Source: CAD feature listing. Evaluate the final solid. Frame: model axes, mm. A direction names the side the tool comes from. Give positions to 0.01 mm unless a question says otherwise; leave off trailing zeros. Write each loop counter-clockwise with the first axis right and the second up, starting at its lowest first coordinate (ties: lowest second). Pieces come first, ordered by that corner, then holes. Notation, with made-up numbers: (-12.75, -19.5) -> (2.25, -19.5) arc R35 ccw to (2.25, 17.5) -> close; hole circle Ø6 at (88.25, -25). An arc over 180 degrees is marked (long way). Write item = value, one per line.
from build123d import *

# Parameters (mm, degrees)
F1_DEPTH       = 12.7
F3_D           = 3.7973
F3_CSINK_D     = 7.7978
F3_CSINK_ANGLE = 82
F4_W           = 8.128
F4_H           = 9.6413786206
F4_H_2         = 9.652
F5_DEPTH       = 25.4
F7_DEPTH       = 12.7
F9_DEPTH       = 25.4
F11_DEPTH      = 25.4


with BuildPart() as f1:
    # F0 (on Right) → F1 (new body, symmetric)
    with BuildSketch(Plane.YZ):
        Polygon((0, 6.35), (0, 31.75), (-3.048, 31.75), (-3.048, 0), (0, 0), (3.175, 6.35), align=None)
    extrude(amount=F1_DEPTH, both=True)

    # F3 (through all)
    with Locations(Plane.XZ.offset(3.048)):
        with Locations((-6.35, 25.4), (6.35, 25.4), (0, 14.224)):
            CounterSinkHole(F3_D / 2, F3_CSINK_D / 2, counter_sink_angle=F3_CSINK_ANGLE)

    # F4 (on face) → F5 (cut)
    with BuildSketch(Plane(origin=(0, 0, 0), x_dir=(-1, 0, 0), z_dir=(0, 1, 0))):
        with Locations((-5.588, -1.5186893103)):
            Rectangle(F4_W, F4_H)
        with Locations((5.588, -1.5133786206)):
            Rectangle(F4_W, F4_H_2)
    extrude(amount=F5_DEPTH, mode=Mode.SUBTRACT)

    # F6 (on Right) → F7 (cut, symmetric)
    with BuildSketch(Plane.YZ):
        with BuildLine():
            Line((-1.4666680983, 4.0132), (-4.4497507624, 4.0132))
            Line((-4.4497507624, 4.0132), (-4.4497507624, 0))
            Line((-4.4497507624, 0), (-2.9257507624, 0))
            Line((-2.9257507624, 0), (-1.0280151601, 3.2489821244))
            ThreePointArc((-1.0280151601, 3.2489821244), (-1.0260874129, 3.7580886308), (-1.4666680983, 4.0132))
        make_face()
    extrude(amount=F7_DEPTH, both=True, mode=Mode.SUBTRACT)

    # F8 (on Front) → F9 (cut)
    with BuildSketch(Plane.XZ):
        Polygon((0.088738686, -6.674986371), (11.087261314, -6.674986371), (5.588, 2.850013629), align=None)
    extrude(amount=F9_DEPTH, mode=Mode.SUBTRACT)

    # F10 (on face) → F11 (cut)
    with BuildSketch(Plane(origin=(0, 0, 0), x_dir=(-1, 0, 0), z_dir=(0, 1, 0))):
        Polygon((0.088738686, -6.6802), (11.087261314, -6.6802), (5.588, 2.8448), align=None)
    extrude(amount=-F11_DEPTH, mode=Mode.SUBTRACT)


solid = f1.part
1) Contact query for flat-ended pins moving along their axis: pin 1 (8 mm diameter, centred on x = -8, z = 4, fed in from +Y) (3 decimals); pin 2 (1.7 mm diameter, centred on x = -5.5, z = 1.5, fed in from +Y); pin 3 (0.5 mm diameter, centred on x = 7, y = 0.5, fed in from -Z). Output: stop coordinate, or through.
Computed:
pin_1 = 3.175
pin_2 = 0
pin_3 = 3.3
2) Material intervals for L1, parallel to X at y = -0.15, z = 25.4; L2, parallel to Z at x = 0, y = -0.6; L3, parallel to Z at x = 9.5, y = -2.5, sorted ascending.
Computed:
L1 = -12.7 to -8.25, -4.45 to 4.45, 8.25 to 12.7
L2 = 0 to 12.33, 16.12 to 31.75
L3 = 0 to 0.73, 4.01 to 24.06, 26.74 to 31.75
3) Cut plane C-C (z = 25.4). Return the cut outline in (x, y), then the cut area to 3 significant figures.
Computed:
outline = (-12.7, -3.05) -> (-10.25, -3.05) -> (-8.25, -0.75) -> (-8.25, 0) -> (-12.7, 0) -> close; (-4.45, -0.75) -> (-2.45, -3.05) -> (2.45, -3.05) -> (4.45, -0.75) -> (4.45, 0) -> (-4.45, 0) -> close; (8.25, -0.75) -> (10.25, -3.05) -> (12.7, -3.05) -> (12.7, 0) -> (8.25, 0) -> close
area = 45.1 mm²
4) Access query for faces 5 (the flat face through (-9.652, 0.4, 2.4)), 6 (the flat face through (0.18, -1.99, 1.6)), 7 (the flat face through (0, 0, 19)). Directions: +Z, -Z, +X, -X, +Y, -Y. A direction counts if a zero-diameter tool reaches every point of the face in a straight line with its end or side. Return the directions, or none.
Computed:
face_5 = -Z, +Y
face_6 = +X, -X, -Y
face_7 = +Z, +X, -X, +Y
5) Cut plane D-D (y = 0.5). Return the cut outline in (x, z), then the cut area to 3 significant figures.
Computed:
outline = (-12.7, 1) -> (-9.65, 1) -> (-9.65, 3.31) -> (-1.52, 3.31) -> (-1.52, 1) -> (1.52, 1) -> (1.52, 3.3) -> (9.65, 3.3) -> (9.65, 1) -> (12.7, 1) -> (12.7, 6.35) -> (-12.7, 6.35) -> close
area = 98.4 mm²
6) Cut plane B-B (x = 0). Return the cut outline in (y, z) (3 decimals), then the cut area to 3 significant figures.
Computed:
outline = (-3.048, 4.013) -> (-1.467, 4.013) arc R0.508 cw to (-1.028, 3.249) -> (-2.926, 0) -> (0, 0) -> (3.175, 6.35) -> (0, 6.35) -> (0, 12.325) -> (-0.747, 12.325) -> (-3.048, 10.325) -> close; (-3.048, 18.123) -> (-0.747, 16.123) -> (0, 16.123) -> (0, 31.75) -> (-3.048, 31.75) -> close
area = 85.7 mm²
7) Cut plane A-A (y = -2). Return the cut outline in (x, z).
Computed:
outline = (-12.7, 0) -> (-7.23, 0) -> (-6.32, 1.58) -> (-12.7, 1.58) -> close; (-12.7, 4.01) -> (12.7, 4.01) -> (12.7, 31.75) -> (-12.7, 31.75) -> close; (-4.86, 1.58) -> (-3.95, 0) -> (3.94, 0) -> (4.86, 1.58) -> close; (6.32, 1.58) -> (7.23, 0) -> (12.7, 0) -> (12.7, 1.58) -> close; hole circle Ø5.98 at (-6.35, 25.4); hole circle Ø5.98 at (0, 14.22); hole circle Ø5.98 at (6.35, 25.4)
8) Draft query along Z for faces 1 (the flat face through (0, -2, 4.013)), 2 (the flat face through (0, -2, 31.75)), 3 (the flat face through (-4.6, 0, 1.7)), 4 (the flat face through (10, -1, 0)). Return one class per face: pulls with the +Z half, pulls with the -Z half, needs draft (parallel to the pull), parting line crosses it, or undercut.
Computed:
face_1 = undercut
face_2 = pulls with the +Z half
face_3 = needs draft
face_4 = pulls with the -Z half
